The model under review builds one solid part; all positions refer to its coordinate system, in mm. Face numbers are marked on the shaded views. A direction names the side the tool comes from. Give positions to 0.01 mm unless a question says otherwise; leave off trailing zeros. Order: outer loops, then holes, each group sorted by start corner. A loop starts at its lowest first (then second) coordinate and runs counter-clockwise, first axis right, second up.
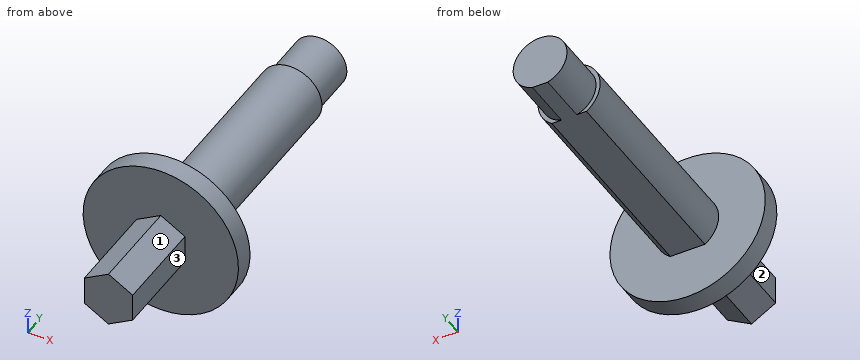
```python
from build123d import *

# Parameters (mm, degrees)
BOSS_EXTRUDE1_DEPTH = 9
BOSS_EXTRUDE2_DEPTH = 22.4
SKETCH3_R           = 7.5
BOSS_EXTRUDE3_DEPTH = 2
BOSS_EXTRUDE4_DEPTH = 5


with BuildPart() as part:
    # Sketch1 → Boss-Extrude1 (new body)
    with BuildSketch(Plane(origin=(0, 0, 0), x_dir=(1, 0, 0), z_dir=(0, 1, 0))):
        Polygon((0, 2.7), (-2.33826859, 1.35), (-2.33826859, -1.35), (0, -2.7), (2.33826859, -1.35), (2.33826859, 1.35), align=None)
    extrude(amount=BOSS_EXTRUDE1_DEPTH)

    # Sketch2 → Boss-Extrude2 (add)
    with BuildSketch(Plane(origin=(0, 9, 0), x_dir=(1, 0, 0), z_dir=(0, 1, 0))):
        with BuildLine():
            Line((-1.667829968, 2.493660602), (1.667829968, 2.493660602))
            ThreePointArc((1.667829968, 2.493660602), (0, -3), (-1.667829968, 2.493660602))
        make_face()
    extrude(amount=BOSS_EXTRUDE2_DEPTH)

    # Sketch3 → Boss-Extrude3 (add)
    with BuildSketch(Plane.XZ.offset(-9)):
        with Locations(Location((0, 0, 0), (0, 0, 270))):
            Circle(SKETCH3_R)
    extrude(amount=-BOSS_EXTRUDE3_DEPTH)

    # Sketch4 → Boss-Extrude4 (add)
    with BuildSketch(Plane(origin=(0, 31.4, 0), x_dir=(1, 0, 0), z_dir=(0, 1, 0))):
        with BuildLine():
            Line((-0.735973371, 2.493660602), (0.735973371, 2.493660602))
            ThreePointArc((0.735973371, 2.493660602), (0, -2.6), (-0.735973371, 2.493660602))
        make_face()
    extrude(amount=BOSS_EXTRUDE4_DEPTH)


solid = part.part
```
Item 1: For line 1 (Y direction, x = 4.5, z = -0.75); line 2 (Y direction, x = -1.5, z = -2.25); line 3 (X direction, y = 32, z = -1.75), list the stretches that pass through material, from the lowest coordinate up.
Values found:
line 1: y = 9 to 11
line 2: y = 9 to 31.4
line 3: x = -1.92 to 1.92
Item 2: Clearance check with flat-ended pins moving along their axes: pin 1 Ø3 at (x, z) = (4, 3.5) entering from -Y; pin 2 Ø5 at (x, y) = (1.5, 24) entering from +Z; pin 3 Ø2.5 at (x, y) = (0, 23) entering from -Z. State where each tip first meets the part, or that it passes through.
Values found:
pin 1: stops at y = 9
pin 2: stops at z = 3
pin 3: stops at z = -2.49
Item 3: Take a section at C-C (z = -6). Give the boundary of the cut face in (x, y), and give its area (3 significant figures).
Values found:
outline: (-4.5, 9) - (4.5, 9) - (4.5, 11) - (-4.5, 11) - close
area: 18.0 mm2
Item 4: Take a section at B-B (z = 0). Give the boundary of the cut face in (x, y).
Values found:
outline: (-7.5, 9) - (-2.34, 9) - (-2.34, 0) - (2.34, 0) - (2.34, 9) - (7.5, 9) - (7.5, 11) - (3, 11) - (3, 31.4) - (2.6, 31.4) - (2.6, 36.4) - (-2.6, 36.4) - (-2.6, 31.4) - (-3, 31.4) - (-3, 11) - (-7.5, 11) - close
Item 5: Take a section at D-D (y = 25.5). Give the boundary of the cut face in (x, z), and give its area (3 significant figures).
Values found:
outline: (-1.67, -2.49) - (1.67, -2.49) arc R3 ccw (long way) to start
area: 27.1 mm2
Item 6: For the marked faces 1, 2 and 3, list the 3-axis set-ups (+Z, -Z, +X, -X, +Y, -Y) from which the entire face can be reached by the end or side of a thin tool; tool diameter is ignored.
Values found:
face 1: +Z, +X, -Y
face 2: +Z, -Z, -X, -Y
face 3: +Z, -Z, +X, -Y
Item 7: Take a section at A-A (y = 2). Give the boundary of the cut face in (x, z).
Values found:
outline: (-2.34, -1.35) - (0, -2.7) - (2.34, -1.35) - (2.34, 1.35) - (0, 2.7) - (-2.34, 1.35) - close
